Study the drawing (mm; zero at the part's minimum x, y, z) and answer. A direction names the side the tool comes from. Give positions to 0.01 mm unless a question says otherwise; leave off trailing zeros. Order: outer loops, then holes, each group sorted by start corner. A loop starts at its lowest first (then second) coordinate and runs counter-clockwise, first axis right, second up.
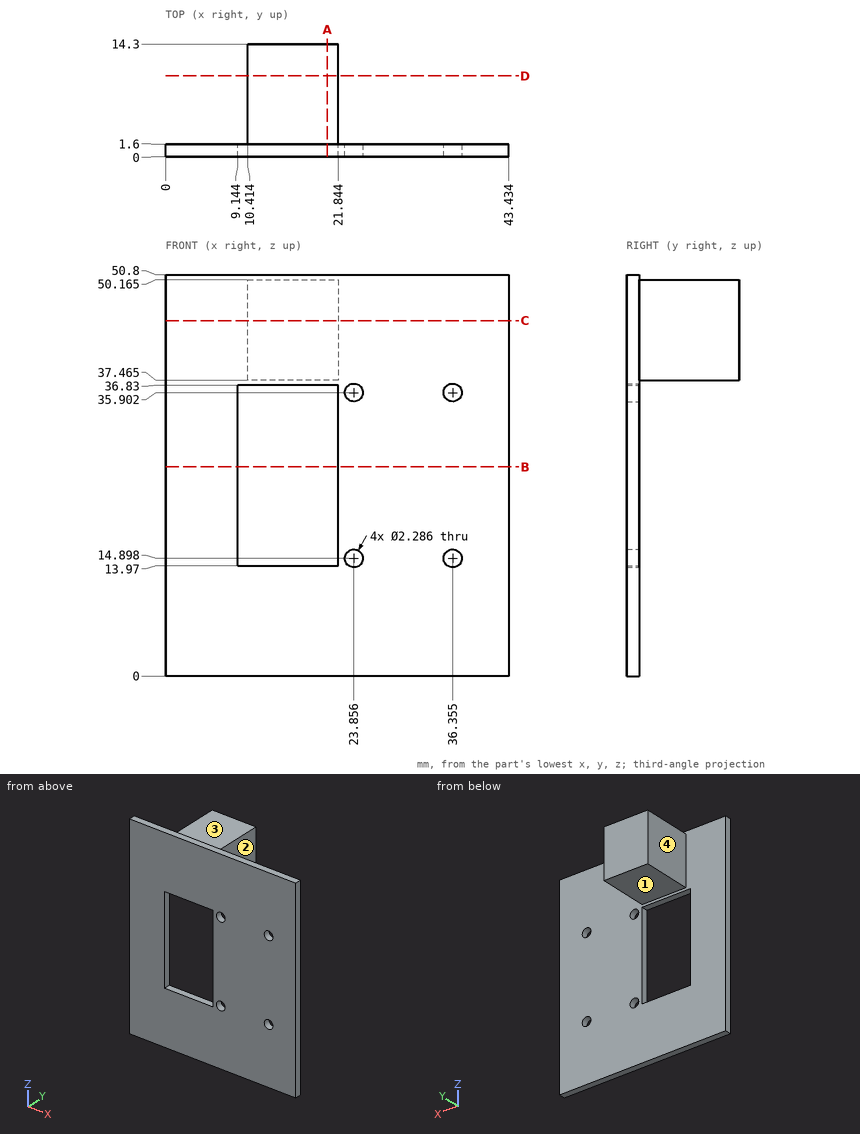
1) Find section C-C (z = 45). Write down the section's boundary in (x, y).
Geometry says:
outline: (0, 0) - (43.43, 0) - (43.43, 1.6) - (21.84, 1.6) - (21.84, 14.3) - (10.41, 14.3) - (10.41, 1.6) - (0, 1.6) - close
2) Find section A-A (x = 20.5). Write down the section's boundary in (y, z) (1 decimal).
Geometry says:
outline: (0, 0) - (1.6, 0) - (1.6, 14) - (0, 14) - close; (0, 36.8) - (1.6, 36.8) - (1.6, 37.5) - (14.3, 37.5) - (14.3, 50.2) - (1.6, 50.2) - (1.6, 50.8) - (0, 50.8) - close
3) Given P1, Ø3.5, axis at x = 36.35, z = 14.9, coming from the -Y side; P2, Ø4, axis at y = 10.5, z = 42.5, coming from the -X side; P3, Ø4, axis at x = 17, y = 8, coming from the +Z side (3 decimals); P4, Ø2, axis at x = 8.5, y = 4.5, coming from the -Z side, each flat-ended and moving along its own axis, determine where each tip first touches the part or whether it passes through.
Geometry says:
P1: stops at y = 0
P2: stops at x = 10.41
P3: stops at z = 50.165
P4: passes through
4) A tool of negligible diameter and unlimited length cuts with its end or side. For the marked faces 1, 2, 3 and 4, from which of +Z, -Z, +X, -X, +Y, -Y can it reach the whole face along a straight path? Write none if from no direction.
Geometry says:
face 1: -Z, +X, -X, +Y
face 2: +Z, -Z, +X, +Y
face 3: +Z, +X, -X, +Y
face 4: +Z, -Z, -X, +Y
5) Find section D-D (y = 10.25). Write down the section's boundary in (x, z) (1 decimal), then the cut area to 3 significant figures.
Geometry says:
outline: (10.4, 37.5) - (21.8, 37.5) - (21.8, 50.2) - (10.4, 50.2) - close
area: 145 mm2
6) Find section B-B (z = 26.5). Write down the section's boundary in (x, y).
Geometry says:
outline: (0, 0) - (9.14, 0) - (9.14, 1.6) - (0, 1.6) - close; (21.84, 0) - (43.43, 0) - (43.43, 1.6) - (21.84, 1.6) - close
7) Straight lines are drawn through the part: probe 1 along X at (y, z) = (7.5, 47); probe 2 along Z at (x, y) = (12, 2) (1 decimal); probe 3 along Y at (x, z) = (19, 7.5). For each, find the intervals that lie inside material, in ascending order.
Geometry says:
probe 1: x = 10.41 to 21.84
probe 2: z = 37.5 to 50.2
probe 3: y = 0 to 1.6
